Check sheet for the modelled part. Datum: model origin and axes. Units: mm. Face numbers are marked on the shaded views. A direction names the side the tool comes from. Coordinates: 2 decimals unless noted, no trailing zeros. Loops run counter-clockwise (first coordinate to the right, second up) from the corner with the lowest first, then second, coordinate; pieces in that order, holes last. Notation, with made-up numbers: M -35,8.25 L -9,8.25 A6 ccw -9,19.25 Z; hole C 46,62 d6. An arc over 180 degrees is marked long. Use CSV: the item, a comma, the result in double quotes. Start each with the question number.
(1) Set-up check for the marked faces 1, 2 and 3: record each of +Z, -Z, +X, -X, +Y, -Y from which the full face is reachable in a straight line by a thin tool's end or side.
(2) Go/stop test with flat-tipped pins: pin 1 Ø1.9 at (x, y) = (-3, 2) entering from -Z; pin 2 Ø3 at (x, y) = (25, 3) entering from -Z; pin 3 Ø3 at (y, z) = (4.5, -31.5) entering from +X. Record where each tip stops, or that it passes through.
(3) Section check A-A on x = -2. Record the cut outline in (y, z).
(4) Scan lines: line 1 (Z direction, x = -3, y = 5.25); line 2 (X direction, y = 1.25, z = -52.5) (3 decimals); line 3 (Z direction, x = 17.5, y = 2.5). Record each from-to range of solid material in increasing order.
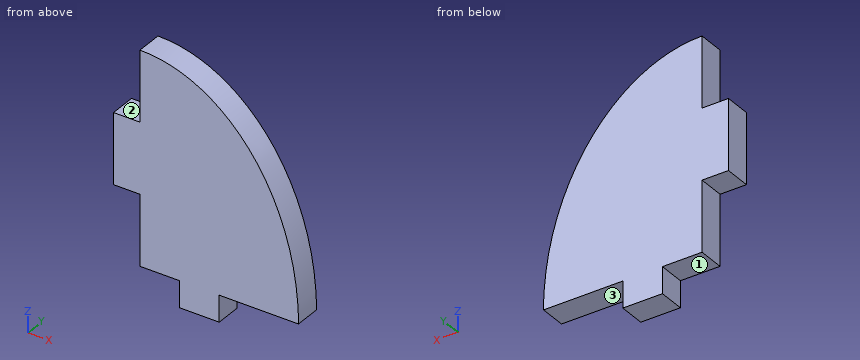
from build123d import *

# Parameters (mm, degrees)
BOSS_EXTRUDE1_DEPTH = 6.35


with BuildPart() as part:
    # Sketch1 → Boss-Extrude1 (new body)
    with BuildSketch(Plane(origin=(0, 0, 0), x_dir=(1, 0, 0), z_dir=(0, 1, 0))):
        with BuildLine():
            Line((0, 0), (0, 16.933333418))
            Line((0, 16.933333418), (-6.35, 16.933333418))
            Line((-6.35, 16.933333418), (-6.35, 33.866666751))
            Line((-6.35, 33.866666751), (0, 33.866666751))
            Line((0, 33.866666751), (0, 50.800000085))
            Line((0, 50.800000085), (9.525, 50.800000085))
            Line((9.525, 50.800000085), (9.525, 57.150000085))
            Line((9.525, 57.150000085), (19.05, 57.150000085))
            Line((19.05, 57.150000085), (19.05, 50.800000085))
            Line((19.05, 50.800000085), (38.1, 50.800000085))
            add(Edge.make_bspline(
                [(0, 0), (38.1, 0), (38.1, 50.800000085)],
                knots=[3.141592654, 3.141592654, 3.141592654, 4.71238898, 4.71238898, 4.71238898], degree=2, weights=[1, 0.707106781, 1]))
        make_face()
    extrude(amount=BOSS_EXTRUDE1_DEPTH)


solid = part.part
Outcome:
1,face 1,"-Z, -X, +Y, -Y"
1,face 2,"+Z, -X, +Y, -Y"
1,face 3,"-Z, +X, +Y, -Y"
2,pin 1,"stops at z = -33.87"
2,pin 2,"stops at z = -50.8"
2,pin 3,"stops at x = 35.68"
3,outline,"M 0,-33.87 L 6.35,-33.87 L 6.35,-16.93 L 0,-16.93 Z"
4,line 1,"z = -33.87 to -16.93"
4,line 2,"x = 9.525 to 19.05"
4,line 3,"z = -57.15 to -5.68"
